Source: CAD feature listing. Evaluate the final solid. Frame: model axes, mm. Face numbers are marked on the shaded views. A direction names the side the tool comes from. Coordinates: 2 decimals unless noted, no trailing zeros. Write each loop counter-clockwise with the first axis right and the second up, starting at its lowest first coordinate (ties: lowest second). Pieces come first, ordered by that corner, then holes. Notation, with made-up numbers: (66, 88.25) - (72, 88.25) arc R26 cw to (72, 114.25) - close; hole circle Ø9 at (8.5, 83.5). An arc over 180 degrees is marked (long way). One line per item, written item: value.
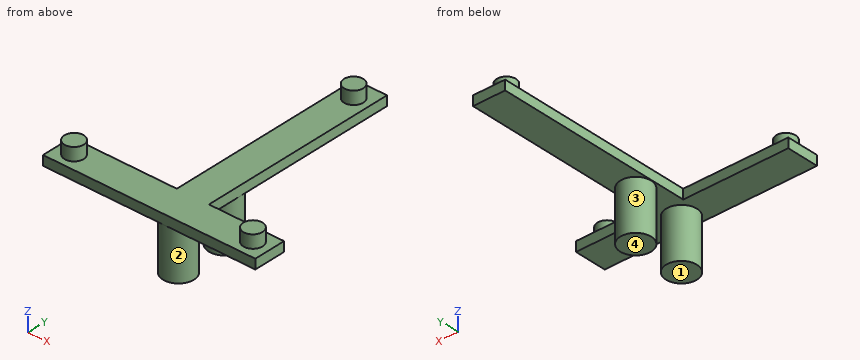
from build123d import *

# Parameters (mm, degrees)
BOSS_EXTRUDE2_DEPTH = 1.5
SKETCH5_R           = 1.5
BOSS_EXTRUDE5_DEPTH = 3.5
SKETCH6_R           = 2.4
BOSS_EXTRUDE6_DEPTH = 7.76


with BuildPart() as part:
    # Sketch4 → Boss-Extrude2 (new body)
    with BuildSketch(Plane.XY):
        Polygon((-139.561248012, 16.070535031), (-106.561248012, 16.070535031), (-106.561248012, 21.070535031), (-118.231248012, 21.070535031), (-118.231248012, 52.070535031), (-123.231248012, 52.070535031), (-123.231248012, 21.070535031), (-139.561248012, 21.070535031), align=None)
    extrude(amount=BOSS_EXTRUDE2_DEPTH)

    # Sketch5 → Boss-Extrude5 (add)
    with BuildSketch(Plane(origin=(0, 0, 0), x_dir=(-1, 0, 0), z_dir=(0, 0, -1))):
        with Locations((136.961248012, 18.570535031)):
            Circle(SKETCH5_R)
        with Locations((109.161248012, 18.570535031)):
            Circle(SKETCH5_R)
        with Locations((120.731248012, 49.070535031)):
            Circle(SKETCH5_R)
    extrude(amount=-BOSS_EXTRUDE5_DEPTH)

    # Sketch6 → Boss-Extrude6 (add)
    with BuildSketch(Plane(origin=(0, 0, 0), x_dir=(-1, 0, 0), z_dir=(0, 0, -1))):
        with Locations((120.731248012, 18.570535031)):
            Circle(SKETCH6_R)
        with Locations((120.731248012, 26.540535031)):
            Circle(SKETCH6_R)
    extrude(amount=BOSS_EXTRUDE6_DEPTH)


solid = part.part
1) Contact query for flat-ended pins moving along their axis: P1, Ø3, axis at x = -118, y = 45, coming from the +Z side; P2, Ø5, axis at y = 48, z = -3, coming from the +X side; P3, Ø2, axis at x = -111, y = 22, coming from the -Z side; P4, Ø0.8, axis at x = -132, z = 1, coming from the +Y side. Output: stop coordinate, or through.
Values found:
P1: z = 1.5
P2: through
P3: z = 0
P4: y = 21.07
2) Draft query along Y for the marked faces 3 and 4. Return one class per face: released by +Y, released by -Y, zero draft, split by the parting line, or undercut.
Values found:
face 3: undercut
face 4: zero draft
3) Section query D-D on z = -3.5. Output: boundary loops of the cut face in (x, y), then the cut area to 3 significant figures.
Values found:
outline: circle Ø4.8 at (-120.73, 18.57); circle Ø4.8 at (-120.73, 26.54)
area: 36.2 mm2
4) Section query A-A on z = 0.5. Output: boundary loops of the cut face in (x, y).
Values found:
outline: (-139.56, 16.07) - (-106.56, 16.07) - (-106.56, 21.07) - (-118.23, 21.07) - (-118.23, 52.07) - (-123.23, 52.07) - (-123.23, 21.07) - (-139.56, 21.07) - close
5) Material intervals for line 1 (X direction, y = 19.5, z = 2.75); line 2 (X direction, y = 27, z = 0.75); line 3 (Z direction, x = -122, y = 43), sorted ascending.
Values found:
line 1: -138.14 to -135.78, -110.34 to -107.98
line 2: -123.23 to -118.23
line 3: 0 to 1.5
6) Reachability of the marked faces 1 and 2 from +Z, -Z, +X, -X, +Y, -Y: full face, straight path, thin tool, end or side. Return the list, or none.
Values found:
face 1: -Z, +X, -X, +Y, -Y
face 2: -Z
7) Section query C-C on x = -114.5. Output: boundary loops of the cut face in (y, z), then the cut area to 3 significant figures.
Values found:
outline: (16.07, 0) - (21.07, 0) - (21.07, 1.5) - (16.07, 1.5) - close
area: 7.50 mm2
8) Section query B-B on y = 48.5. Output: boundary loops of the cut face in (x, z), then the cut area to 3 significant figures.
Values found:
outline: (-123.23, 0) - (-118.23, 0) - (-118.23, 1.5) - (-119.34, 1.5) - (-119.34, 3.5) - (-122.12, 3.5) - (-122.12, 1.5) - (-123.23, 1.5) - close
area: 13.0 mm2
